Source: CAD feature listing. Evaluate the final solid. Frame: model axes, mm. Face numbers are marked on the shaded views. A direction names the side the tool comes from. Give positions to 0.01 mm unless a question says otherwise; leave off trailing zeros. Write each loop counter-clockwise with the first axis right and the second up, starting at its lowest first coordinate (ties: lowest second). Pieces come first, ordered by that corner, then holes. Notation, with made-up numbers: M 18,71 L 33,71 A35 ccw 33,109 Z; hole C -15,-20 d10. An arc over 180 degrees is marked long. Return JSON: item names as keys, results as strings.
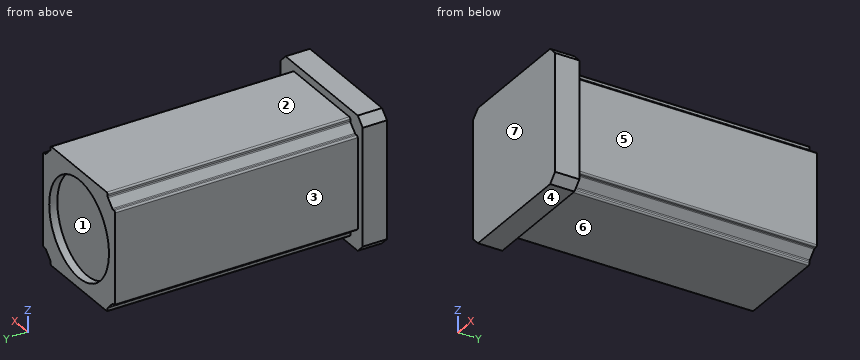
```python
from build123d import *

# Parameters (mm, degrees)
BOSS_EXTRUDE1_DEPTH = 30
BOSS_EXTRUDE2_DEPTH = 300
SKETCH3_R           = 60
CUT_EXTRUDE1_DEPTH  = 10
FILLET1_R           = 2


with BuildPart() as part:
    # Sketch1 → Boss-Extrude1 (new body)
    with BuildSketch(Plane(origin=(0, 0, 0), x_dir=(1, 0, 0), z_dir=(0, 1, 0))):
        Polygon((-82.5, 72.5), (-72.5, 82.5), (72.5, 82.5), (82.5, 72.5), (82.5, -72.5), (72.5, -82.5), (-72.5, -82.5), (-82.5, -72.5), align=None)
    extrude(amount=BOSS_EXTRUDE1_DEPTH)

    # Sketch2 → Boss-Extrude2 (add)
    with BuildSketch(Plane(origin=(0, 30, 0), x_dir=(1, 0, 0), z_dir=(0, 1, 0))):
        Polygon((72.5, 57.5), (67.5, 57.5), (57.5, 67.5), (57.5, 72.5), (-57.5, 72.5), (-57.5, 67.5), (-67.5, 57.5), (-72.5, 57.5), (-72.5, -57.5), (-67.5, -57.5), (-57.5, -67.5), (-57.5, -72.5), (57.5, -72.5), (57.5, -67.5), (67.5, -57.5), (72.5, -57.5), align=None)
    extrude(amount=BOSS_EXTRUDE2_DEPTH)

    # Sketch3 → Cut-Extrude1 (cut)
    with BuildSketch(Plane(origin=(0, 330, 0), x_dir=(1, 0, 0), z_dir=(0, 1, 0))):
        Circle(SKETCH3_R)
    extrude(amount=-CUT_EXTRUDE1_DEPTH, mode=Mode.SUBTRACT)

    # Fillet1
    fillet1_edges = [part.edges().sort_by_distance(p)[0] for p in [
        (72.5, 180, 57.5),
        (72.5, 180, -57.5),
        (67.5, 180, -57.5),
        (57.5, 180, -67.5),
        (57.5, 180, -72.5),
        (-57.5, 180, -72.5),
        (-57.5, 180, -67.5),
        (-67.5, 180, -57.5),
        (-72.5, 180, -57.5),
        (-72.5, 180, 57.5),
        (-67.5, 180, 57.5),
        (-57.5, 180, 67.5),
        (-57.5, 180, 72.5),
        (57.5, 180, 72.5),
        (57.5, 180, 67.5),
        (67.5, 180, 57.5),
    ]]
    fillet(fillet1_edges, radius=FILLET1_R)


solid = part.part
```
1) Draft query along Z for the marked faces 1, 2, 3 and 4. Return one class per face: released by +Z, released by -Z, zero draft, split by the parting line, or undercut.
Numbers:
{"face 1": "undercut", "face 2": "released by +Z", "face 3": "zero draft", "face 4": "released by -Z"}
2) Line query: line 1 (X direction, y = 327.25, z = 0); line 2 (Y direction, x = 7, z = -35). Output: solid intervals per line, ascending. Write a range as [from, to].
Numbers:
{"line 1": "x = [-72.5, -60], [60, 72.5]", "line 2": "y = [0, 320]"}
3) Cut plane B-B, the plane z = 0. Return the cut outline in (x, y), then the cut area to 4 significant figures.
Numbers:
{"outline": "M -82.5,0 L 82.5,0 L 82.5,30 L 72.5,30 L 72.5,330 L 60,330 L 60,320 L -60,320 L -60,330 L -72.5,330 L -72.5,30 L -82.5,30 Z", "area": "47,250 mm²"}
4) Contact query for flat-ended pins moving along their axis: pin 1 Ø6 at (x, y) = (45, 139.5) entering from -Z; pin 2 Ø4 at (y, z) = (39.5, 30) entering from +X; pin 3 Ø1.1 at (x, y) = (69.5, 193) entering from +Z. Output: stop coordinate, or through.
Numbers:
{"pin 1": "stops at z = -72.5", "pin 2": "stops at x = 72.5", "pin 3": "stops at z = 57.5"}
5) Set-up query: the marked faces 5, 6 and 7. Return all of +Z, -Z, +X, -X, +Y, -Y with unobstructed straight access to the full face (end or side cutting, diameter ignored); none if empty.
Numbers:
{"face 5": "+Z, -Z, +X, +Y", "face 6": "-Z, +X, -X, +Y", "face 7": "+Z, -Z, +X, -X, -Y"}
6) Cut plane A-A, the plane x = 0. Return the cut outline in (y, z), then the cut area to 4 significant figures.
Numbers:
{"outline": "M 0,-82.5 L 30,-82.5 L 30,-72.5 L 330,-72.5 L 330,-60 L 320,-60 L 320,60 L 330,60 L 330,72.5 L 30,72.5 L 30,82.5 L 0,82.5 Z", "area": "47,250 mm²"}
